Verification items for the finished model (mm, model axes). Face numbers are marked on the shaded views. A direction names the side the tool comes from. Coordinates: 2 decimals unless noted, no trailing zeros. Loops run counter-clockwise (first coordinate to the right, second up) from the corner with the lowest first, then second, coordinate; pieces in that order, holes last. Notation, with made-up numbers: (62, 64.5) - (101, 64.5) arc R26 ccw to (101, 102.5) - close; hole circle Ø6 at (41.25, 82.5). An arc over 180 degrees is marked (long way). One line per item, written item: value. Start each with the question number.
(1) Set-up check for the marked faces 1, 2, 3, 4 and 5: record each of +Z, -Z, +X, -X, +Y, -Y from which the full face is reachable in a straight line by a thin tool's end or side.
(2) Section check A-A (x = 0). Record the boundary of the cut face in (y, z), plus the area to 3 significant figures.
(3) Section check B-B (z = -99.5). Record the boundary of the cut face in (x, y), plus the area to 3 significant figures.
(4) Section check D-D (x = -107). Record the boundary of the cut face in (y, z).
(5) Section check C-C (y = -27). Record the boundary of the cut face in (x, z), plus the area to 3 significant figures.
(6) Draft check along Y on the marked faces 6, 7, 8 and 9. Enter one of: +Y half, -Y half, draft (parallel to the pull), parting line (faces both ways), or undercut.
(7) Gauge pin test, flat ends, axial feed: P1, Ø24, axis at y = -11, z = -7.5, coming from the -X side; P2, Ø13.5, axis at x = -111, y = 0, coming from the -Z side; P3, Ø1, axis at y = -18.5, z = 53.5, coming from the +X side. Record the tip position at first contact, or that the pin passes through.
(8) Thickness scan on probe 1 along X at (y, z) = (-9, -29); probe 2 along X at (y, z) = (-19, -47); probe 3 along Z at (x, y) = (94.5, -20.5). Record the ranges inside material, lowest first. Write a range as [from, to].
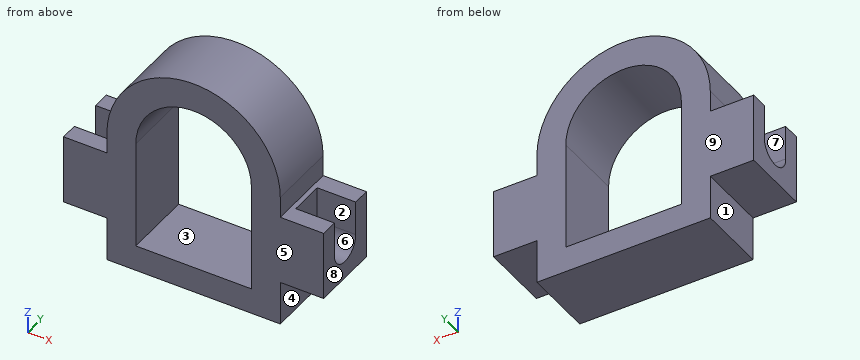
```python
from build123d import *

# Parameters (mm, degrees)
F1_DEPTH = 36
F2_W     = 40
F2_H     = 36
F5_DEPTH = 36
F6_DEPTH = 40
F7_DEPTH = 40


with BuildPart() as f1:
    # F0 (on Front) → F1 (new body, symmetric)
    with BuildSketch(Plane.XZ):
        with BuildLine():
            Line((90, -22), (90, 0))
            ThreePointArc((90, 0), (0, 90), (-90, 0))
            Line((-90, 0), (-90, -22))
            Line((-90, -22), (-135, -22))
            Line((-135, -22), (-135, -94))
            Line((-135, -94), (-90, -94))
            Line((-90, -94), (-90, -140))
            Line((-90, -140), (90, -140))
            Line((90, -140), (90, -94))
            Line((90, -94), (135, -94))
            Line((135, -94), (135, -22))
            Line((135, -22), (90, -22))
        make_face()
        with BuildLine():
            ThreePointArc((-60, 0), (0, 60), (60, 0))
            Line((60, 0), (60, -113))
            Line((60, -113), (-60, -113))
            Line((-60, -113), (-60, 0))
        make_face(mode=Mode.SUBTRACT)
    extrude(amount=F1_DEPTH, both=True)

    # F2 (on face) → F5 (cut)
    with BuildSketch(Plane.XY.offset(-22)):
        with Locations((-115, 0)):
            Rectangle(F2_W, F2_H)
        with Locations((115, 0)):
            Rectangle(F2_W, F2_H)
    extrude(amount=-F5_DEPTH, mode=Mode.SUBTRACT)

    # F3 (on face) → F6 (cut)
    with BuildSketch(Plane(origin=(-135, 0, 0), x_dir=(0, -1, 0), z_dir=(-1, 0, 0))):
        with BuildLine():
            Line((18, -58), (-18, -58))
            ThreePointArc((-18, -58), (0, -76), (18, -58))
        make_face()
    extrude(amount=-F6_DEPTH, mode=Mode.SUBTRACT)

    # F4 (on face) → F7 (cut)
    with BuildSketch(Plane.YZ.offset(135)):
        with BuildLine():
            ThreePointArc((-18, -58), (0, -76), (18, -58))
            Line((18, -58), (-18, -58))
        make_face()
    extrude(amount=-F7_DEPTH, mode=Mode.SUBTRACT)


solid = f1.part
```
Responses:
1. face 1: -Z, -X, +Y, -Y
1. face 2: +Z, +X
1. face 3: +Y, -Y
1. face 4: -Z, +X, +Y, -Y
1. face 5: +Z, -Z, +X, -X, -Y
2. outline: (-36, -140) - (36, -140) - (36, -113) - (-36, -113) - close; (-36, 60) - (36, 60) - (36, 90) - (-36, 90) - close
2. area: 4,100 mm²
3. outline: (-90, -36) - (-60, -36) - (-60, 36) - (-90, 36) - close; (60, -36) - (90, -36) - (90, 36) - (60, 36) - close
3. area: 4,320 mm²
4. outline: (-36, -94) - (36, -94) - (36, -22) - (18, -22) - (18, -58) arc R18 cw to (-18, -58) - (-18, -22) - (-36, -22) - close
5. outline: (-135, -94) - (-90, -94) - (-90, -140) - (90, -140) - (90, -94) - (135, -94) - (135, -22) - (90, -22) - (90, 0) arc R90 ccw to (-90, 0) - (-90, -22) - (-135, -22) - close; hole (-60, -113) - (60, -113) - (60, 0) arc R60 ccw to (-60, 0) - close
5. area: 25,200 mm²
6. face 6: undercut
6. face 7: undercut
6. face 8: draft
6. face 9: +Y half
7. P1: stops at x = -90
7. P2: stops at z = -94
7. P3: stops at x = 72.74
8. probe 1: x = [-95, -60], [60, 95]
8. probe 2: x = [-135, -60], [60, 135]
8. probe 3: z = [-94, -22]
